Model file for the job. Use its own axes, mm. Face numbers are marked on the shaded views. Coordinates: 2 decimals unless noted, no trailing zeros. Write each loop counter-clockwise with the first axis right and the second up, starting at its lowest first coordinate (ties: lowest second). Pieces come first, ordered by that corner, then holes.
Q1. Pin check, flat tips, straight feed: P1, Ø1.5, axis at y = 8.5, z = -7.5, coming from the +X side; P2, Ø3, axis at y = 13, z = -12.5, coming from the -X side; P3, Ø5, axis at y = 13, z = -5.5, coming from the +X side. Stop position of each tip, or through.
Q2. Band-saw the part on A-A, the plane x = 0. Write the cut outline in (y, z).
Q3. Band-saw the part on C-C, the plane z = -8. Write the cut outline in (x, y), plus the area to 3 significant figures.
Q4. Pull direction X, two halves, no side cores. Call the marked faces 1, 2 and 3: released by +X, released by -X, zero draft, split by the parting line, or undercut.
Q5. Band-saw the part on B-B, the plane y = 3.81. State how many separate pieces and enclosed holes the cut face has, plus the area to 3 significant figures.
Q6. Drill centre lines: probe 1 along Y at (x, z) = (-21, 0); probe 2 along X at (y, z) = (10, -1.5); probe 3 along Z at (x, y) = (-4, 23). Where is each one in solid material? Low to high.
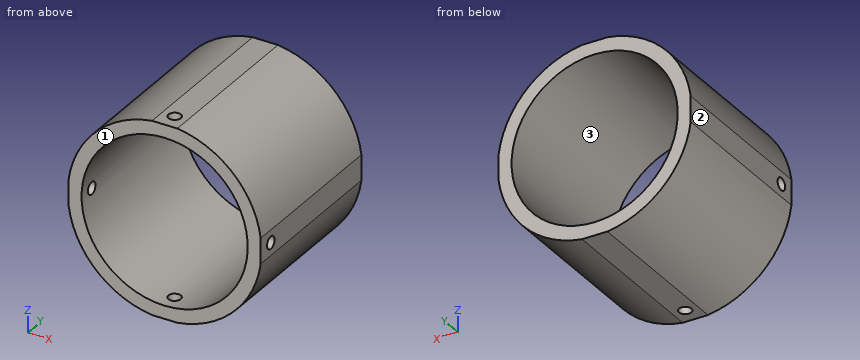
from build123d import *

# Parameters (mm, degrees)
SKETCH1_R               = 22.225
SKETCH1_R_2             = 19.05
BOSS_EXTRUDE1_DEPTH     = 38.1
CUT_EXTRUDE1_DEPTH      = 43.18
CUT_EXTRUDE1_DEPTH_BACK = 43.18
SKETCH2_R               = 1.4224
CUT_EXTRUDE2_DEPTH      = 43.18
CUT_EXTRUDE2_DEPTH_BACK = 43.18
SKETCH3_R               = 1.4224
SKETCH4_W               = 49.025527768
SKETCH4_H               = 48.000320082
SKETCH4_W_2             = 44.069
SKETCH4_H_2             = 44.069
CUT_EXTRUDE3_DEPTH      = 43.18


with BuildPart() as part:
    # Sketch1 → Boss-Extrude1 (new body)
    with BuildSketch(Plane(origin=(0, 0, 0), x_dir=(1, 0, 0), z_dir=(0, 1, 0))):
        with Locations(Location((0, 0, 0), (0, 0, 90))):
            Circle(SKETCH1_R)
        with Locations(Location((0, 0, 0), (0, 0, 90))):
            Circle(SKETCH1_R_2, mode=Mode.SUBTRACT)
    extrude(amount=BOSS_EXTRUDE1_DEPTH)

    # Sketch2 → Cut-Extrude1 (cut, two sides: drawn at the far end of the back side and taken through both)
    with BuildSketch(Plane.XY.offset(-CUT_EXTRUDE1_DEPTH_BACK)):
        with Locations(Location((0, 3.81, 0), (0, 0, 180))):
            Circle(SKETCH2_R)
    extrude(amount=CUT_EXTRUDE1_DEPTH + CUT_EXTRUDE1_DEPTH_BACK, mode=Mode.SUBTRACT)

    # Sketch3 → Cut-Extrude2 (cut, two sides: drawn at the far end of the back side and taken through both)
    with BuildSketch(Plane(origin=(0, 0, 0), x_dir=(0, 0, -1), z_dir=(1, 0, 0)).offset(-CUT_EXTRUDE2_DEPTH_BACK)):
        with Locations(Location((0, 3.81, 0), (0, 0, 180))):
            Circle(SKETCH3_R)
    extrude(amount=CUT_EXTRUDE2_DEPTH + CUT_EXTRUDE2_DEPTH_BACK, mode=Mode.SUBTRACT)

    # Sketch4 → Cut-Extrude3 (cut)
    with BuildSketch(Plane.XZ):
        Rectangle(SKETCH4_W, SKETCH4_H)
        Rectangle(SKETCH4_W_2, SKETCH4_H_2, mode=Mode.SUBTRACT)
    extrude(amount=-CUT_EXTRUDE3_DEPTH, mode=Mode.SUBTRACT)


solid = part.part
Answer sheet:
1. P1: stops at x = 21.18
1. P2: stops at x = -19.31
1. P3: stops at x = 22.02
2. outline: (0, -22.03) - (2.39, -22.03) - (2.39, -19.05) - (0, -19.05) - close; (0, 19.05) - (2.39, 19.05) - (2.39, 22.03) - (0, 22.03) - close; (5.23, -22.03) - (38.1, -22.03) - (38.1, -19.05) - (5.23, -19.05) - close; (5.23, 19.05) - (38.1, 19.05) - (38.1, 22.03) - (5.23, 22.03) - close
3. outline: (-20.74, 0) - (-17.29, 0) - (-17.29, 38.1) - (-20.74, 38.1) - close; (17.29, 0) - (20.74, 0) - (20.74, 38.1) - (17.29, 38.1) - close
3. area: 263 mm2
4. face 1: zero draft
4. face 2: released by -X
4. face 3: undercut
5. separate pieces: 4
5. enclosed holes: 0
5. area: 375 mm2
6. probe 1: y = 0 to 2.39, 5.23 to 38.1
6. probe 2: x = -22.03 to -18.99, 18.99 to 22.03
6. probe 3: z = -21.86 to -18.63, 18.63 to 21.86
